Geometry check sheet. Reference: the model listing, model coordinates, mm. A direction names the side the tool comes from. Round coordinates to 2 decimals unless told otherwise and drop trailing zeros. Order: outer loops, then holes, each group sorted by start corner. A loop starts at its lowest first (then second) coordinate and runs counter-clockwise, first axis right, second up.
(1) Set-up check for faces 4 (the face through (0, -27, 2)), 5 (the face through (0, -2, 5)): record each of +Z, -Z, +X, -X, +Y, -Y from which the full face is reachable in a straight line by a thin tool's end or side.
(2) Go/stop test with flat-tipped pins: pin 1 (12 mm diameter, centred on x = -16.5, z = 35.5, fed in from -Y); pin 2 (10 mm diameter, centred on x = -15, y = -9.5, fed in from +Z). Record where each tip stops, or that it passes through.
(3) Sectioned sample at C-C (z = 59.37). Record the boundary of the cut face in (x, y), plus the area to 3 significant figures.
(4) Release check for a two-part mould opening along X. For faces 1 (the face through (-27, 24, 19)), 2 (the face through (11.264, 17.338, 2.465)), 3 (the face through (0, 23, 37)) record: +X half, -X half, draft (parallel to the pull), parting line (faces both ways), or undercut.
(5) Sectioned sample at B-B (y = 20). Record the boundary of the cut face in (x, z).
(6) Material ranges on line 1 along X through (y, z) = (24.95, 59.37); line 2 along Z through (x, y) = (3.5, -2.5); line 3 along X through (y, z) = (-20, 3.65), recorded low to high.
(7) Sectioned sample at D-D (x = 12). Record the boundary of the cut face in (y, z).
(8) Sectioned sample at A-A (x = -20). Record the boundary of the cut face in (y, z).
from build123d import *

# Parameters (mm, degrees)
ESQUISSE1_W             = 54
ESQUISSE1_H             = 54
ESQUISSE1_R             = 3
BOSS_EXTRU_1_DEPTH      = 67.37
ESQUISSE2_W             = 85.887974464
ESQUISSE2_H             = 58.790343592
ENL_V_MAT_EXTRU_1_DEPTH = 62.37
ESQUISSE3_R             = 3
ENL_V_MAT_EXTRU_2_DEPTH = 62.37


with BuildPart() as part:
    # Esquisse1 → Boss.-Extru.1 (new body)
    with BuildSketch(Plane.XY):
        Rectangle(ESQUISSE1_W, ESQUISSE1_H)
        with Locations((9.88, 20)):
            Circle(ESQUISSE1_R, mode=Mode.SUBTRACT)
        with Locations((9.88, -20)):
            Circle(ESQUISSE1_R, mode=Mode.SUBTRACT)
    extrude(amount=BOSS_EXTRU_1_DEPTH)

    # Esquisse2 → Enlèv. mat.-Extru.1 (cut)
    with BuildSketch(Plane.XY.offset(67.37)):
        with Locations((-4.168944697, -6.395171796)):
            Rectangle(ESQUISSE2_W, ESQUISSE2_H)
    extrude(amount=-ENL_V_MAT_EXTRU_1_DEPTH, mode=Mode.SUBTRACT)

    # Esquisse3 → Enlèv. mat.-Extru.2 (cut)
    with BuildSketch(Plane.XZ.offset(-23)):
        with Locations(Location((-20, 59.37, 0), (0, 0, 270))):
            Circle(ESQUISSE3_R)
        with Locations(Location((20, 59.37, 0), (0, 0, 270))):
            Circle(ESQUISSE3_R)
    extrude(amount=-ENL_V_MAT_EXTRU_2_DEPTH, mode=Mode.SUBTRACT)


solid = part.part
Answer below:
1. face 4: +Z, -Z, +X, -X, -Y
1. face 5: +Z, +X, -X, -Y
2. pin 1: stops at y = 23
2. pin 2: stops at z = 5
3. outline: (-27, 23) - (-23, 23) - (-23, 27) - (-27, 27) - close; (-17, 23) - (17, 23) - (17, 27) - (-17, 27) - close; (23, 23) - (27, 23) - (27, 27) - (23, 27) - close
3. area: 168 mm2
4. face 1: -X half
4. face 2: undercut
4. face 3: draft
5. outline: (-27, 0) - (6.88, 0) - (6.88, 5) - (-27, 5) - close; (12.88, 0) - (27, 0) - (27, 5) - (12.88, 5) - close
6. line 1: x = -27 to -23, -17 to 17, 23 to 27
6. line 2: z = 0 to 5
6. line 3: x = -27 to 6.88, 12.88 to 27
7. outline: (-27, 0) - (-22.12, 0) - (-22.12, 5) - (-27, 5) - close; (-17.88, 0) - (17.88, 0) - (17.88, 5) - (-17.88, 5) - close; (22.12, 0) - (27, 0) - (27, 67.37) - (23, 67.37) - (23, 5) - (22.12, 5) - close
8. outline: (-27, 0) - (27, 0) - (27, 56.37) - (23, 56.37) - (23, 5) - (-27, 5) - close; (23, 62.37) - (27, 62.37) - (27, 67.37) - (23, 67.37) - close
